The model under review builds one solid part; all positions refer to its coordinate system, in mm. A direction names the side the tool comes from. Coordinates: 2 decimals unless noted, no trailing zeros. Order: outer loops, then holes, each group sorted by start corner. A loop starts at its lowest first (then second) coordinate and runs counter-clockwise, first axis right, second up. Notation, with made-up numbers: M -5.5,82 L 45.5,82 A21 cw 45.5,89 Z; hole C 56,72.25 d8. An arc over 180 degrees is marked long. Answer as CSV lines item,"result". Start each with the question number.
Q1. Machinability: for faces 5 (the face through (30.38, 1.45, -1.43)), 6 (the face through (1.1, 27.54, -58.93)), 7 (the face through (58.9, 27.54, -1.07)), which of the approach directions +Z, -Z, +X, -X, +Y, -Y give a long, thin tool a straight path to every point of the face, cutting with its end or side? Answer none if there is none.
Q2. Consider section D-D on y = 27.25. Write out the cut boundary in (x, z), and give its area (3 significant figures).
Q3. Consider section B-B on z = -23. Write out the cut boundary in (x, y), and give its area (3 significant figures).
Q4. Consider section A-A on y = 8.75. Write out the cut boundary in (x, z), and give its area (3 significant figures).
Q5. The part is to be moulded in two halves that separate along Z. For faces 1 (the face through (58.57, 1.45, -30.38)), 2 (the face through (30, 14, -60)), 3 (the face through (30, 16, -1)), 4 (the face through (59.5, 28, -30)), say which applies: +Z half, -Z half, draft (parallel to the pull), parting line (faces both ways), or undercut.
Q6. Wall thickness on L1, parallel to X at y = 19.5, z = -3; L2, parallel to Z at x = 48.5, y = 17; L3, parallel to Z at x = 12.5, y = 27.75: over which ranges is each line inside the solid? List them lowest first. Write a range as [from, to].
Q7. For P1, Ø1.5, axis at y = 27, z = -38, coming from the -X side; P2, Ø4, axis at x = 6, z = -51.5, coming from the +Y side; P3, Ø2.5, axis at x = 41.5, y = 27, coming from the +Z side, all flat-tipped, find the tip position at first contact; note any pin that passes through.
Q8. Consider section C-C on x = 42. Write out the cut boundary in (y, z).
from build123d import *

# Parameters (mm, degrees)
SKETCH1_W           = 60
SKETCH1_H           = 60
BOSS_EXTRUDE1_DEPTH = 25
FILLET1_R           = 2.5
SHELL1_T            = -1
BOSS_EXTRUDE2_START = 5
BOSS_EXTRUDE2_DEPTH = 5


with BuildPart() as part:
    # Sketch1 → Boss-Extrude1 (new body)
    with BuildSketch(Plane(origin=(0, 0, 0), x_dir=(1, 0, 0), z_dir=(0, 1, 0))):
        with Locations((30, 30)):
            Rectangle(SKETCH1_W, SKETCH1_H)
    extrude(amount=BOSS_EXTRUDE1_DEPTH)

    # Fillet1
    fillet1_edges = [part.edges().sort_by_distance(p)[0] for p in [
        (30, 0, -60),
        (60, 0, -30),
        (30, 0, 0),
        (0, 0, -30),
        (0, 12.5, -60),
        (60, 12.5, -60),
        (60, 12.5, 0),
        (0, 12.5, 0),
    ]]
    fillet(fillet1_edges, radius=FILLET1_R)

    # Shell1
    shell1_openings = [part.faces().sort_by_distance(p)[0] for p in [
        (30, 25, -30),
    ]]
    offset(amount=SHELL1_T, openings=shell1_openings, kind=Kind.INTERSECTION)

    # Sketch5 → Boss-Extrude2 (add)
    with BuildSketch(Plane(origin=(0, 25, 0), x_dir=(1, 0, 0), z_dir=(0, 1, 0)).offset(BOSS_EXTRUDE2_START)):
        with BuildLine():
            Line((57.5, 59.5), (2.5, 59.5))
            ThreePointArc((2.5, 59.5), (1.085786438, 58.914213562), (0.5, 57.5))
            Line((0.5, 57.5), (0.5, 2.5))
            ThreePointArc((0.5, 2.5), (1.085786438, 1.085786438), (2.5, 0.5))
            Line((2.5, 0.5), (57.5, 0.5))
            ThreePointArc((57.5, 0.5), (58.914213562, 1.085786438), (59.5, 2.5))
            Line((59.5, 2.5), (59.5, 57.5))
            ThreePointArc((59.5, 57.5), (58.914213562, 58.914213562), (57.5, 59.5))
        make_face()
        with BuildLine():
            Line((57.5, 59), (2.5, 59))
            ThreePointArc((2.5, 59), (1.439339828, 58.560660172), (1, 57.5))
            Line((1, 57.5), (1, 2.5))
            ThreePointArc((1, 2.5), (1.439339828, 1.439339828), (2.5, 1))
            Line((2.5, 1), (57.5, 1))
            ThreePointArc((57.5, 1), (58.560660172, 1.439339828), (59, 2.5))
            Line((59, 2.5), (59, 57.5))
            ThreePointArc((59, 57.5), (58.560660172, 58.560660172), (57.5, 59))
        make_face(mode=Mode.SUBTRACT)
    extrude(amount=-BOSS_EXTRUDE2_DEPTH)


solid = part.part
Evaluation:
1,face 5,"+Y"
1,face 6,"-Z, -X, +Y"
1,face 7,"+Z, +X, +Y"
2,outline,"M 0.5,-57.5 A2 ccw 2.5,-59.5 L 57.5,-59.5 A2 ccw 59.5,-57.5 L 59.5,-2.5 A2 ccw 57.5,-0.5 L 2.5,-0.5 A2 ccw 0.5,-2.5 Z; hole M 1,-57.5 A1.5 ccw 2.5,-59 L 57.5,-59 A1.5 ccw 59,-57.5 L 59,-2.5 A1.5 ccw 57.5,-1 L 2.5,-1 A1.5 ccw 1,-2.5 Z"
2,area,"115 mm²"
3,outline,"M 0,2.5 A2.5 ccw 2.5,0 L 57.5,0 A2.5 ccw 60,2.5 L 60,25 L 59.5,25 L 59.5,30 L 59,30 L 59,2.5 A1.5 cw 57.5,1 L 2.5,1 A1.5 cw 1,2.5 L 1,30 L 0.5,30 L 0.5,25 L 0,25 Z"
3,area,"111 mm²"
4,outline,"M 0,-57.5 A2.5 ccw 2.5,-60 L 57.5,-60 A2.5 ccw 60,-57.5 L 60,-2.5 A2.5 ccw 57.5,0 L 2.5,0 A2.5 ccw 0,-2.5 Z; hole M 1,-57.5 A1.5 ccw 2.5,-59 L 57.5,-59 A1.5 ccw 59,-57.5 L 59,-2.5 A1.5 ccw 57.5,-1 L 2.5,-1 A1.5 ccw 1,-2.5 Z"
4,area,"233 mm²"
5,face 1,"undercut"
5,face 2,"-Z half"
5,face 3,"undercut"
5,face 4,"draft"
6,L1,"x = [0, 1], [59, 60]"
6,L2,"z = [-60, -59], [-1, 0]"
6,L3,"z = [-59.5, -59], [-1, -0.5]"
7,P1,"stops at x = 0.5"
7,P2,"stops at y = 1"
7,P3,"stops at z = -0.5"
8,outline,"M 0,-57.5 A2.5 ccw 2.5,-60 L 25,-60 L 25,-59.5 L 30,-59.5 L 30,-59 L 2.5,-59 A1.5 cw 1,-57.5 L 1,-2.5 A1.5 cw 2.5,-1 L 30,-1 L 30,-0.5 L 25,-0.5 L 25,0 L 2.5,0 A2.5 ccw 0,-2.5 Z"
